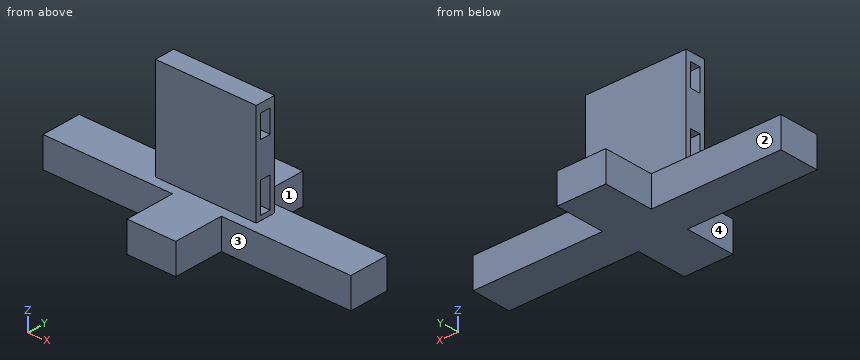
```python
from build123d import *

# Parameters (mm, degrees)
F0_W     = 64.2762212083
F0_H     = 19.7247266769
F0_W_2   = 24.1831187159
F0_H_2   = 24.8195268214
F1_DEPTH = 15
F2_W     = 50
F2_H     = 10
F3_DEPTH = 50
F4_W     = 2.6052840985
F4_H     = 15.0249563158
F4_W_2   = 2.6046917774
F4_H_2   = 11.2548321486
F5_DEPTH = 100


with BuildPart() as f1:
    # F0 (on Top) → F1 (new body)
    with BuildSketch(Plane.XY):
        with Locations((44.2296699621, 0)):
            Rectangle(F0_W, F0_H)
        Rectangle(F0_W_2, F0_H)
        with Locations((0, 22.2721267492)):
            Rectangle(F0_W_2, F0_H_2)
        with Locations((-44.2296699621, 0)):
            Rectangle(F0_W, F0_H)
        with Locations((0, -22.2721267492)):
            Rectangle(F0_W_2, F0_H_2)
    extrude(amount=F1_DEPTH)

    # F2 (on face) → F3 (join)
    with BuildSketch(Plane.XY.offset(15)):
        Rectangle(F2_W, F2_H)
    extrude(amount=F3_DEPTH)

    # F4 (on face) → F5 (cut)
    with BuildSketch(Plane.YZ.offset(25)):
        with Locations((1.3026420493, 24.7752834111)):
            Rectangle(F4_W, F4_H)
        with Locations((-1.3026420493, 24.7752834111)):
            Rectangle(F4_W, F4_H)
        with Locations((-1.3023458887, 55.1106519997)):
            Rectangle(F4_W_2, F4_H_2)
        with Locations((1.3023458887, 55.1106519997)):
            Rectangle(F4_W_2, F4_H_2)
    extrude(amount=-F5_DEPTH, mode=Mode.SUBTRACT)


solid = f1.part
```
Design review of the part built by this model. Coordinates are the model's own, in mm. Face numbers are marked on the shaded views. A direction names the side the tool comes from. Coordinates: 2 decimals unless noted, no trailing zeros. Order: outer loops, then holes, each group sorted by start corner. A loop starts at its lowest first (then second) coordinate and runs counter-clockwise, first axis right, second up. Notation, with made-up numbers: M 87,82 L 118,82 A20 ccw 118,118 Z; hole C 3.25,62.5 d9. An arc over 180 degrees is marked long. Answer as a JSON object with one key per item and string values. Group by question number.
1) Add section A-A, the plane z = 23.5. Write out the cut boundary in (x, y).
2) For pin 1 (4 mm diameter, centred on y = 0.5, z = 49, fed in from -X); pin 2 (5 mm diameter, centred on y = 1.5, z = 34.5, fed in from +X); pin 3 (7.5 mm diameter, centred on x = 32.5, z = 9.5, fed in from -Y), all flat-tipped, find the tip position at first contact; note any pin that passes through.
3) Wall thickness on L1, parallel to Y at x = 18, z = 51.5; L2, parallel to Y at x = -3, z = 15.5; L3, parallel to Y at x = 26, z = 12.5: over which ranges is each line inside the solid? List them lowest first.
4) Add section D-D, the plane z = 58. Write out the cut boundary in (x, y).
5) Tool access review of the marked faces 1, 2, 3 and 4: name each direction out of +Z, -Z, +X, -X, +Y, -Y from which nothing blocks a thin tool from reaching the whole face with its end or side.
6) Add section C-C, the plane x = 22.5. Write out the cut boundary in (y, z).
7) Add section B-B, the plane y = 1. Write out the cut boundary in (x, z).
Computed values:
{
 "1": {"outline": "M -25,-5 L 25,-5 L 25,-2.61 L -25,-2.61 Z; M -25,2.61 L 25,2.61 L 25,5 L -25,5 Z"},
 "2": {"pin 1": "stops at x = -25", "pin 2": "stops at x = 25", "pin 3": "stops at y = -9.86"},
 "3": {"L1": "y = -5 to -2.6, 2.6 to 5", "L2": "y = -5 to 5", "L3": "y = -9.86 to 9.86"},
 "4": {"outline": "M -25,-5 L 25,-5 L 25,-2.6 L -25,-2.6 Z; M -25,2.6 L 25,2.6 L 25,5 L -25,5 Z"},
 "5": {"face 1": "+Z, -Z, +X, +Y", "face 2": "+Z, -Z, -X, +Y", "face 3": "+Z, -Z, +X, -Y", "face 4": "+Z, -Z, -X, -Y"},
 "6": {"outline": "M -9.86,0 L 9.86,0 L 9.86,15 L 5,15 L 5,65 L -5,65 L -5,15 L -9.86,15 Z; hole M -2.61,17.26 L 2.61,17.26 L 2.61,32.29 L -2.61,32.29 Z; hole M -2.6,49.48 L 2.6,49.48 L 2.6,60.74 L -2.6,60.74 Z"},
 "7": {"outline": "M -76.37,0 L 76.37,0 L 76.37,15 L 25,15 L 25,17.26 L -25,17.26 L -25,15 L -76.37,15 Z; M -25,32.29 L 25,32.29 L 25,49.48 L -25,49.48 Z; M -25,60.74 L 25,60.74 L 25,65 L -25,65 Z"}
}
